```python
from build123d import *

# Parameters (mm, degrees)
F2_DEPTH = 30
F3_DEPTH = 30


with BuildPart() as f2:
    # F0 (on Top) → F2 (new body)
    with BuildSketch(Plane.XY):
        with BuildLine():
            ThreePointArc((-0.619784, 0.422336), (-0.716707, 0.220977), (-0.75, 0))
            Line((-0.75, 0), (-0.75, -6.95))
            ThreePointArc((-0.75, -6.95), (0, -7.7), (0.75, -6.95))
            Line((0.75, -6.95), (0.75, -0.231242))
            Line((0.75, -0.231242), (1.886792, 1.437017))
            ThreePointArc((1.886792, 1.437017), (1.689343, 2.479137), (0.647223, 2.281688))
            Line((0.647223, 2.281688), (-0.619784, 0.422336))
        make_face()
    extrude(amount=F2_DEPTH)

    # F1 (on Top) → F3 (join, through all)
    with BuildSketch(Plane.XY):
        with BuildLine():
            Line((-1.45, -17.95), (-1.45, -7.95))
            Line((-1.45, -7.95), (-0.75, -6.95))
            Line((-0.75, -6.95), (-0.75, -4.33431))
            Line((-0.75, -4.33431), (-2.95, -7.477167))
            Line((-2.95, -7.477167), (-2.95, -17.95))
            ThreePointArc((-2.95, -17.95), (-2.2, -18.7), (-1.45, -17.95))
        make_face()
    extrude(amount=F3_DEPTH)


solid = f2.part
```
Here's how the part is built. I have some questions about the finished solid (model axes, mm). A direction names the side the tool comes from. Coordinates: 2 decimals unless noted, no trailing zeros. Write each loop counter-clockwise with the first axis right and the second up, starting at its lowest first coordinate (ties: lowest second). Pieces come first, ordered by that corner, then holes. Notation, with made-up numbers: (-26, -12) - (21, -12) arc R10 ccw to (21, 4) - close; hole circle Ø8 at (35, 67.25). An arc over 180 degrees is marked (long way). One line per item, written item: value.
1) On a 3-axis mill with a long thin cutter (end or side, diameter ignored), from which of +Z, -Z, +X, -X, +Y, -Y can I reach the whole of each face in a straight line? I mean faces 4 (the flat face through (-1.45, -13, 15)), 5 (the flat face through (-1.83, -5.88, 14.79)). Say none if no direction works.
Model answer:
face 4: +Z, -Z, +X, -Y
face 5: +Z, -Z, -X, +Y
2) Suppose I cut it at C-C on x = 0.1. Write out the boundary of the cut face in (y, z).
Model answer:
outline: (-7.69, 0) - (1.48, 0) - (1.48, 30) - (-7.69, 30) - close
3) Suppose I cut it at B-B on y = -3.5. Write out the boundary of the cut face in (x, z), and give its area (3 significant figures).
Model answer:
outline: (-0.75, 0) - (0.75, 0) - (0.75, 30) - (-0.75, 30) - close
area: 45.0 mm²
4) We'd pull the mould along X, two halves only. Please class faces 1 (the cylindrical face through (0, -7.7, 14.8)), 2 (the flat face through (-1, -7, 0)), 3 (the flat face through (-0.75, -2, 15)): pulls with the +X half, pulls with the -X half, needs draft (parallel to the pull), parting line crosses it, or undercut.
Model answer:
face 1: undercut
face 2: needs draft
face 3: pulls with the -X half
5) I need wall thicknesses on line 1 along X through (y, z) = (-10.75, 9.5); line 2 along X through (y, z) = (-0.5, 5.5); line 3 along Y through (x, z) = (-1.65, 28). Which ranges of each line are inside material? Lowest first, please.
Model answer:
line 1: x = -2.95 to -1.45
line 2: x = -0.75 to 0.75
line 3: y = -18.46 to -5.62
6) Suppose I cut it at A-A on z = 22.5. Write out the boundary of the cut face in (x, y).
Model answer:
outline: (-2.95, -17.95) arc R0.75 ccw to (-1.45, -17.95) - (-1.45, -7.95) - (-0.75, -6.95) arc R0.75 ccw to (0.75, -6.95) - (0.75, -0.23) - (1.89, 1.44) arc R0.75 ccw to (0.65, 2.28) - (-0.62, 0.42) arc R0.75 ccw to (-0.75, 0) - (-0.75, -4.33) - (-2.95, -7.48) - close
7) I'm going to push flat-ended pins straight in: P1, Ø1, axis at x = -2, z = 4, coming from the +Y side; P2, Ø5, axis at y = -1.5, z = 17, coming from the -X side; P3, Ø4, axis at y = -11.5, z = 14, coming from the +X side. Where does each tip first touch, or does it pass through?
Model answer:
P1: stops at y = -5.41
P2: stops at x = -0.75
P3: stops at x = -1.45
